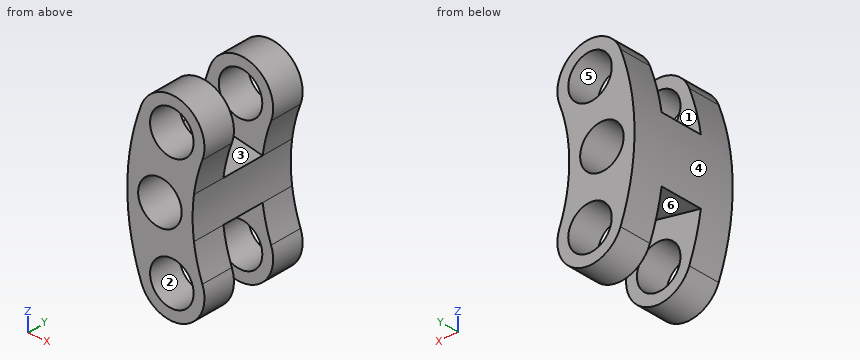
from build123d import *

# Parameters (mm, degrees)
F0_R     = 5
F1_DEPTH = 12.5
F2_DEPTH = 5


# Not quite as in the source:
# - a feature of the source that left no trace in its solid (it failed there, or was rolled back) is left out


with BuildPart() as f1:
    # F0 (on Front) → F1 (new body, symmetric)
    with BuildSketch(Plane.XZ):
        with BuildLine():
            ThreePointArc((5.0784583206, 4.6742255002), (5.8300100803, 8.5686007088), (7.0173413473, 12.3529411765))
            ThreePointArc((7.0173413473, 12.3529411765), (2.6470588235, 22.0173413473), (-7.0173413473, 17.6470588235))
            ThreePointArc((-7.0173413473, 17.6470588235), (-8.6271086588, 12.5781627487), (-9.6893672694, 7.3669570477))
            Line((-9.6893672694, 7.3669570477), (5.0784583206, 4.6742255002))
        make_face()
        with Locations((0, 15)):
            Circle(F0_R, mode=Mode.SUBTRACT)
        with BuildLine():
            ThreePointArc((5.0784583206, -4.6742255002), (4.7649343015, 0), (5.0784583206, 4.6742255002))
            Line((5.0784583206, 4.6742255002), (-9.6893672694, 7.3669570477))
            ThreePointArc((-9.6893672694, 7.3669570477), (-10.2350656985, 0), (-9.6893672694, -7.3669570477))
            Line((-9.6893672694, -7.3669570477), (5.0784583206, -4.6742255002))
        make_face()
        with Locations((-2.7350656985, 0)):
            Circle(F0_R, mode=Mode.SUBTRACT)
        with BuildLine():
            ThreePointArc((7.0173413473, -12.3529411765), (5.8300100803, -8.5686007088), (5.0784583206, -4.6742255002))
            Line((5.0784583206, -4.6742255002), (-9.6893672694, -7.3669570477))
            ThreePointArc((-9.6893672694, -7.3669570477), (-8.6271086588, -12.5781627487), (-7.0173413473, -17.6470588235))
            ThreePointArc((-7.0173413473, -17.6470588235), (2.6470588235, -22.0173413473), (7.0173413473, -12.3529411765))
        make_face()
        with Locations((0, -15)):
            Circle(F0_R, mode=Mode.SUBTRACT)
    extrude(amount=F1_DEPTH, both=True)

    # F0 (on Front) → F2 (cut, symmetric)
    with BuildSketch(Plane.XZ):
        with BuildLine():
            ThreePointArc((5.0784583206, 4.6742255002), (5.8300100803, 8.5686007088), (7.0173413473, 12.3529411765))
            ThreePointArc((7.0173413473, 12.3529411765), (2.6470588235, 22.0173413473), (-7.0173413473, 17.6470588235))
            ThreePointArc((-7.0173413473, 17.6470588235), (-8.6271086588, 12.5781627487), (-9.6893672694, 7.3669570477))
            Line((-9.6893672694, 7.3669570477), (5.0784583206, 4.6742255002))
        make_face()
        with Locations((0, 15)):
            Circle(F0_R, mode=Mode.SUBTRACT)
        with BuildLine():
            ThreePointArc((7.0173413473, -12.3529411765), (5.8300100803, -8.5686007088), (5.0784583206, -4.6742255002))
            Line((5.0784583206, -4.6742255002), (-9.6893672694, -7.3669570477))
            ThreePointArc((-9.6893672694, -7.3669570477), (-8.6271086588, -12.5781627487), (-7.0173413473, -17.6470588235))
            ThreePointArc((-7.0173413473, -17.6470588235), (2.6470588235, -22.0173413473), (7.0173413473, -12.3529411765))
        make_face()
        with Locations((0, -15)):
            Circle(F0_R, mode=Mode.SUBTRACT)
    extrude(amount=F2_DEPTH, both=True, mode=Mode.SUBTRACT)


solid = f1.part
For this review, take the finished solid that the model builds, in its own axes (mm). Face numbers are marked on the shaded views. A direction names the side the tool comes from. Round coordinates to 2 decimals unless told otherwise and drop trailing zeros. Write each loop counter-clockwise with the first axis right and the second up, starting at its lowest first coordinate (ties: lowest second). Pieces come first, ordered by that corner, then holes. Notation, with made-up numbers: (70.25, 32.5) - (86.25, 32.5) arc R24 cw to (86.25, 65.5) - close; hole circle Ø6 at (-10, 77.25). An arc over 180 degrees is marked (long way). Use a Markdown table: item, result.
Q1. We need section A-A (z = 0). Give the boundary of the cut face in (x, y), plus the area to 3 significant figures.
Derived:
| item | result |
|---|---|
| outline | (-10.24, -12.5) - (-7.74, -12.5) - (-7.74, 12.5) - (-10.24, 12.5) - close; (2.26, -12.5) - (4.76, -12.5) - (4.76, 12.5) - (2.26, 12.5) - close |
| area | 125 mm2 |
Q2. The part is to be moulded in two halves that separate along X. For the marked faces 1, 2, 3 and 4, say which applies: pulls with the +X half, pulls with the -X half, needs draft (parallel to the pull), parting line crosses it, or undercut.
Derived:
| item | result |
|---|---|
| face 1 | needs draft |
| face 2 | undercut |
| face 3 | pulls with the +X half |
| face 4 | pulls with the -X half |
Q3. Clearance check with flat-ended pins moving along their axes: pin 1 (1 mm diameter, centred on x = 3, y = -1.5, fed in from +Z); pin 2 (6 mm diameter, centred on x = 0, z = 15, fed in from -Y); pin 3 (3 mm diameter, centred on x = -1.5, y = -2.5, fed in from +Z); pin 4 (1 mm diameter, centred on y = -7, z = -3.5, fed in from +X). State where each tip first meets the part, or that it passes through.
Derived:
| item | result |
|---|---|
| pin 1 | stops at z = 5.14 |
| pin 2 | passes through |
| pin 3 | stops at z = 6.15 |
| pin 4 | stops at x = 4.99 |
Q4. We need section B-B (y = -9). Give the boundary of the cut face in (x, z).
Derived:
| item | result |
|---|---|
| outline | (-7.02, -17.65) arc R7.5 ccw to (7.02, -12.35) arc R35 cw to (7.02, 12.35) arc R7.5 ccw to (-7.02, 17.65) arc R50 ccw to start; hole circle Ø10 at (-2.74, 0); hole circle Ø10 at (0, -15); hole circle Ø10 at (0, 15) |
Q5. Machinability: for the marked faces 5 and 6, which of the approach directions +Z, -Z, +X, -X, +Y, -Y give a long, thin tool a straight path to every point of the face, cutting with its end or side? Answer none if there is none.
Derived:
| item | result |
|---|---|
| face 5 | +Y, -Y |
| face 6 | -Z, +X |
Q6. We need section D-D (x = 0). State how many separate pieces and enclosed holes the cut face has, plus the area to 3 significant figures.
Derived:
| item | result |
|---|---|
| separate pieces | 6 |
| enclosed holes | 0 |
| area | 278 mm2 |
Q7. Wall thickness on line 1 along Y through (x, z) = (-6.5, -16.5); line 2 along Z through (x, y) = (-2, -7.75); line 3 along Z through (x, y) = (0, 10.25): over which ranges is each line inside the solid? List them lowest first.
Derived:
| item | result |
|---|---|
| line 1 | y = -12.5 to -5, 5 to 12.5 |
| line 2 | z = -22.23 to -19.58, -10.42 to -4.95, 4.95 to 10.42, 19.58 to 22.23 |
| line 3 | z = -22.5 to -20, -10 to -4.19, 4.19 to 10, 20 to 22.5 |
Q8. We need section C-C (x = 3.5). Give the boundary of the cut face in (y, z).
Derived:
| item | result |
|---|---|
| outline | (-12.5, -21.63) - (-5, -21.63) - (-5, -18.57) - (-12.5, -18.57) - close; (-12.5, -11.43) - (-5, -11.43) - (-5, -4.96) - (5, -4.96) - (5, -11.43) - (12.5, -11.43) - (12.5, 11.43) - (5, 11.43) - (5, 4.96) - (-5, 4.96) - (-5, 11.43) - (-12.5, 11.43) - close; (-12.5, 18.57) - (-5, 18.57) - (-5, 21.63) - (-12.5, 21.63) - close; (5, -21.63) - (12.5, -21.63) - (12.5, -18.57) - (5, -18.57) - close; (5, 18.57) - (12.5, 18.57) - (12.5, 21.63) - (5, 21.63) - close |
